from build123d import *

# Parameters (mm, degrees)
SKETCH001_W  = 0.48
SKETCH001_H  = 0.38
PAD001_DEPTH = 5
PAD_DEPTH    = 8


with BuildPart() as pad001:
    # Sketch001 → Pad001 (new body)
    with BuildSketch(Plane.XY.offset(2.5)):
        Rectangle(SKETCH001_W, SKETCH001_H)
        with Locations((2.54, 0)):
            Rectangle(SKETCH001_W, SKETCH001_H)
    extrude(amount=-PAD001_DEPTH)


with BuildPart() as to_92l_2_narrow:
    # Sketch → Pad (new body)
    with BuildSketch(Plane.XY.offset(2.5)):
        with BuildLine():
            Line((-0.704842, -1.45), (3.244842, -1.45))
            ThreePointArc((3.244842, -1.45), (1.27, 2.45), (-0.704842, -1.45))
        make_face()
    extrude(amount=PAD_DEPTH)

    add(pad001.part)


solid = to_92l_2_narrow.part
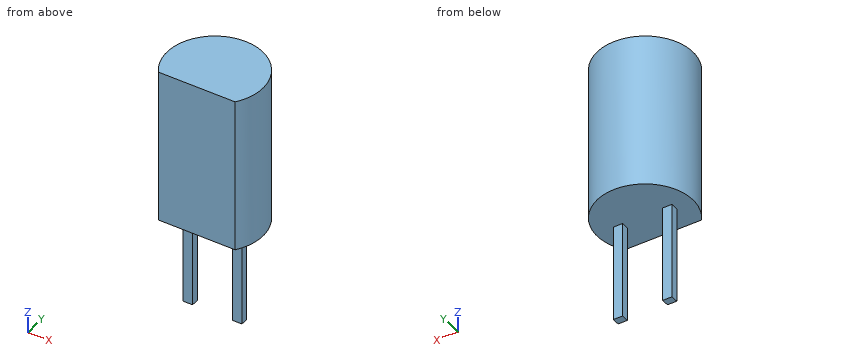
The model under review builds one solid part; all positions refer to its coordinate system, in mm. Coordinates: 2 decimals unless noted, no trailing zeros. Write each loop counter-clockwise with the first axis right and the second up, starting at its lowest first coordinate (ties: lowest second). Pieces come first, ordered by that corner, then holes. Notation, with made-up numbers: (56, -37.75) - (69, -37.75) arc R31 ccw to (69, -13.75) - close; hole circle Ø3 at (-36.5, -11.5). An arc over 180 degrees is marked (long way). Answer as a JSON object with one key per item and string values. Group by question number.
1. Add section C-C (x = 0.1). Give the boundary of the cut face in (y, z).
2. Add section D-D (z = 8.25). Give the boundary of the cut face in (x, y).
3. Add section B-B (y = 0). Give the boundary of the cut face in (x, z), plus the area to 3 significant figures.
4. To check wall thickness, follow probe 1 along Y at (x, z) = (-0.2, 1); probe 2 along Z at (x, y) = (3.4, -0.2); probe 3 along Y at (x, z) = (1.35, 2.75). State the ranges of each line that lie inside material, in increasing order.
5. Clearance check with a flat-ended pin moving along its axis: pin 1 Ø1.2 at (x, y) = (2, 1) entering from -Z. State where the tip first meets the part, or that it passes through.
6. Add section A-A (z = 0.25). Give the boundary of the cut face in (x, y).
Findings:
{
 "1": {"outline": "(-1.45, 2.5) - (-0.19, 2.5) - (-0.19, -2.5) - (0.19, -2.5) - (0.19, 2.5) - (2.15, 2.5) - (2.15, 10.5) - (-1.45, 10.5) - close"},
 "2": {"outline": "(-0.7, -1.45) - (3.24, -1.45) arc R2.45 ccw (long way) to start"},
 "3": {"outline": "(-1.18, 2.5) - (-0.24, 2.5) - (-0.24, -2.5) - (0.24, -2.5) - (0.24, 2.5) - (2.3, 2.5) - (2.3, -2.5) - (2.78, -2.5) - (2.78, 2.5) - (3.72, 2.5) - (3.72, 10.5) - (-1.18, 10.5) - close", "area": "44.0 mm²"},
 "4": {"probe 1": "-0.19 to 0.19", "probe 2": "2.5 to 10.5", "probe 3": "-1.45 to 2.45"},
 "5": {"pin 1": "z = 2.5"},
 "6": {"outline": "(-0.24, -0.19) - (0.24, -0.19) - (0.24, 0.19) - (-0.24, 0.19) - close; (2.3, -0.19) - (2.78, -0.19) - (2.78, 0.19) - (2.3, 0.19) - close"}
}
